The listing builds one solid part. Answer for the finished solid, in the listing's coordinates (mm). Face numbers are marked on the shaded views. A direction names the side the tool comes from. Give positions to 0.01 mm unless a question says otherwise; leave off trailing zeros.
Item 1: Each of these flat-tipped pins is pushed along its axis until it touches: pin 1 Ø1 at (y, z) = (3.5, 4.5) entering from +X; pin 2 Ø1 at (x, z) = (2, 6) entering from +Y; pin 3 Ø4 at (x, y) = (3, 4.5) entering from +Z; pin 4 Ø2 at (x, z) = (3.5, 7) entering from -Y. Where does it stop, or does it pass through?
Item 2: Consider line 1 along X through (y, z) = (6.75, 4.75); line 2 along Z through (x, y) = (3.75, 0.25); line 3 along X through (y, z) = (0.5, 7). Determine where each line is inside the solid, lowest interval first.
Item 3: A tool of negligible diameter and unlimited length cuts with its end or side. For the marked faces 1, 2 and 3, from which of +Z, -Z, +X, -X, +Y, -Y can it reach the whole face along a straight path? Write none if from no direction.
from build123d import *

# Parameters (mm, degrees)
SKETCH2_R           = 1.9
BOSS_EXTRUDE1_DEPTH = 10
SKETCH2_3_R         = 6.5
BOSS_EXTRUDE2_DEPTH = 5
BOSS_EXTRUDE3_DEPTH = 5


with BuildPart() as part:
    # Sketch2 → Boss-Extrude1 (new body)
    with BuildSketch(Plane.XY):
        Circle(SKETCH2_R)
    extrude(amount=BOSS_EXTRUDE1_DEPTH)

    # Sketch2<3> → Boss-Extrude2 (add)
    with BuildSketch(Plane.XY):
        Circle(SKETCH2_3_R)
    extrude(amount=BOSS_EXTRUDE2_DEPTH)

    # Sketch3 → Boss-Extrude3 (add)
    with BuildSketch(Plane(origin=(0, 0, 0), x_dir=(-1, 0, 0), z_dir=(0, 0, -1))):
        with BuildLine():
            Line((0.483224011, 7.501099556), (1.474668872, 7.370573364))
            Line((1.474668872, 7.370573364), (1.682323793, 6.278517871))
            ThreePointArc((1.682323793, 6.278517871), (0.848420249, 6.444391599), (0, 6.5))
            Line((0, 6.5), (0.483224011, 7.501099556))
        make_face()
        with BuildLine():
            Line((3.019609183, 6.883455555), (2.223130932, 6.108002035))
            ThreePointArc((2.223130932, 6.108002035), (3.001365986, 5.765570416), (3.728246836, 5.324488288))
            Line((3.728246836, 5.324488288), (3.906620016, 6.421706942))
            Line((3.906620016, 6.421706942), (3.019609183, 6.883455555))
        make_face()
        with BuildLine():
            Line((5.191784922, 5.435565226), (4.178119463, 4.97928888))
            ThreePointArc((4.178119463, 4.97928888), (4.792302689, 4.39133635), (5.324488288, 3.728246836))
            Line((5.324488288, 3.728246836), (5.86737513, 4.698287889))
            Line((5.86737513, 4.698287889), (5.191784922, 5.435565226))
        make_face()
        with BuildLine():
            Line((6.737754778, 3.332065509), (5.629165125, 3.25))
            ThreePointArc((5.629165125, 3.25), (6.005216961, 2.48744231), (6.278517871, 1.682323793))
            Line((6.278517871, 1.682323793), (7.12043821, 2.408185976))
            Line((7.12043821, 2.408185976), (6.737754778, 3.332065509))
        make_face()
        with BuildLine():
            Line((7.471051968, 0.826669516), (6.401250395, 1.128713155))
            ThreePointArc((6.401250395, 1.128713155), (6.49381344, 0.283526018), (6.475265538, -0.566512328))
            Line((6.475265538, -0.566512328), (7.514671356, -0.172378706))
            Line((7.514671356, -0.172378706), (7.471051968, 0.826669516))
        make_face()
        with BuildLine():
            Line((7.30323003, -1.778435021), (6.401250395, -1.128713155))
            ThreePointArc((6.401250395, -1.128713155), (6.19916018, -1.954587697), (5.891000616, -2.747018701))
            Line((5.891000616, -2.747018701), (7.002524231, -2.732151972))
            Line((7.002524231, -2.732151972), (7.30323003, -1.778435021))
        make_face()
        with BuildLine():
            Line((6.254530767, -4.169034047), (5.629165125, -3.25))
            ThreePointArc((5.629165125, -3.25), (5.156796712, -3.956949289), (4.596194078, -4.596194078))
            Line((4.596194078, -4.596194078), (5.645769338, -4.962387388))
            Line((5.645769338, -4.962387388), (6.254530767, -4.169034047))
        make_face()
        with BuildLine():
            Line((4.451442786, -6.056786039), (4.178119463, -4.97928888))
            ThreePointArc((4.178119463, -4.97928888), (3.492447454, -5.482044398), (2.747018701, -5.891000616))
            Line((2.747018701, -5.891000616), (3.60805134, -6.594085648))
            Line((3.60805134, -6.594085648), (4.451442786, -6.056786039))
        make_face()
        with BuildLine():
            Line((2.111445108, -7.214000246), (2.223130932, -6.108002035))
            ThreePointArc((2.223130932, -6.108002035), (1.406857491, -6.345924046), (0.566512328, -6.475265538))
            Line((0.566512328, -6.475265538), (1.135149101, -7.43043986))
            Line((1.135149101, -7.43043986), (2.111445108, -7.214000246))
        make_face()
        with BuildLine():
            Line((-0.483224011, -7.501099556), (0, -6.5))
            ThreePointArc((0, -6.5), (-0.848420249, -6.444391599), (-1.682323793, -6.278517871))
            Line((-1.682323793, -6.278517871), (-1.474668872, -7.370573364))
            Line((-1.474668872, -7.370573364), (-0.483224011, -7.501099556))
        make_face()
        with BuildLine():
            Line((-3.019609183, -6.883455555), (-2.223130932, -6.108002035))
            ThreePointArc((-2.223130932, -6.108002035), (-3.001365986, -5.765570416), (-3.728246836, -5.324488288))
            Line((-3.728246836, -5.324488288), (-3.906620016, -6.421706942))
            Line((-3.906620016, -6.421706942), (-3.019609183, -6.883455555))
        make_face()
        with BuildLine():
            Line((-5.191784922, -5.435565226), (-4.178119463, -4.97928888))
            ThreePointArc((-4.178119463, -4.97928888), (-4.792302689, -4.39133635), (-5.324488288, -3.728246836))
            Line((-5.324488288, -3.728246836), (-5.86737513, -4.698287889))
            Line((-5.86737513, -4.698287889), (-5.191784922, -5.435565226))
        make_face()
        with BuildLine():
            Line((-6.737754778, -3.332065509), (-5.629165125, -3.25))
            ThreePointArc((-5.629165125, -3.25), (-6.005216961, -2.48744231), (-6.278517871, -1.682323793))
            Line((-6.278517871, -1.682323793), (-7.12043821, -2.408185976))
            Line((-7.12043821, -2.408185976), (-6.737754778, -3.332065509))
        make_face()
        with BuildLine():
            Line((-7.471051968, -0.826669516), (-6.401250395, -1.128713155))
            ThreePointArc((-6.401250395, -1.128713155), (-6.49381344, -0.283526018), (-6.475265538, 0.566512328))
            Line((-6.475265538, 0.566512328), (-7.514671356, 0.172378706))
            Line((-7.514671356, 0.172378706), (-7.471051968, -0.826669516))
        make_face()
        with BuildLine():
            Line((-7.30323003, 1.778435021), (-6.401250395, 1.128713155))
            ThreePointArc((-6.401250395, 1.128713155), (-6.19916018, 1.954587697), (-5.891000616, 2.747018701))
            Line((-5.891000616, 2.747018701), (-7.002524231, 2.732151972))
            Line((-7.002524231, 2.732151972), (-7.30323003, 1.778435021))
        make_face()
        with BuildLine():
            Line((-6.254530767, 4.169034047), (-5.629165125, 3.25))
            ThreePointArc((-5.629165125, 3.25), (-5.156796712, 3.956949289), (-4.596194078, 4.596194078))
            Line((-4.596194078, 4.596194078), (-5.645769338, 4.962387388))
            Line((-5.645769338, 4.962387388), (-6.254530767, 4.169034047))
        make_face()
        with BuildLine():
            Line((-4.451442786, 6.056786039), (-4.178119463, 4.97928888))
            ThreePointArc((-4.178119463, 4.97928888), (-3.492447454, 5.482044398), (-2.747018701, 5.891000616))
            Line((-2.747018701, 5.891000616), (-3.60805134, 6.594085648))
            Line((-3.60805134, 6.594085648), (-4.451442786, 6.056786039))
        make_face()
        with BuildLine():
            Line((-2.111445108, 7.214000246), (-2.223130932, 6.108002035))
            ThreePointArc((-2.223130932, 6.108002035), (-1.406857491, 6.345924046), (-0.566512328, 6.475265538))
            Line((-0.566512328, 6.475265538), (-1.135149101, 7.43043986))
            Line((-1.135149101, 7.43043986), (-2.111445108, 7.214000246))
        make_face()
    extrude(amount=-BOSS_EXTRUDE3_DEPTH)


solid = part.part
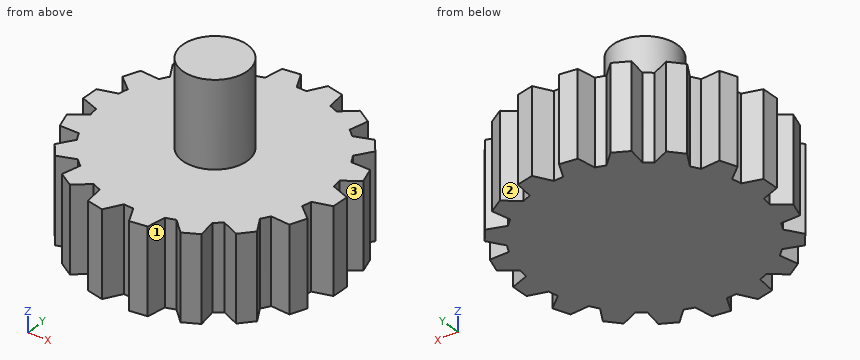
Worked answers:
1. pin 1: stops at x = 6.14
1. pin 2: stops at y = 1.17
1. pin 3: stops at z = 5
1. pin 4: passes through
2. line 1: x = -3.28 to -2.88, -1.59 to -0.12, 0.73 to 2.16
2. line 2: z = 0 to 5
2. line 3: x = -1.83 to 1.83
3. face 1: +Z, -Z, -Y
3. face 2: +Z, -Z, +Y
3. face 3: +Z, -Z, +X
